```python
from build123d import *

# Parameters (mm, degrees)
F0_W     = 146.05
F0_H     = 114.3
F0_R     = 3.24
F0_W_2   = 5
F1_DEPTH = 50
F2_W     = 119.824
F2_H     = 108.7
F3_DEPTH = 45
F4_D     = 5.6
F4_DEPTH = 20
F4_TIP   = 1.6824097333
F5_W     = 40
F5_H     = 5
F6_DEPTH = 2.8
F7_D     = 4
F8_W     = 40
F8_H     = 10
F9_DEPTH = 50.001
F10_R    = 4


with BuildPart() as f1:
    # F0 (on Top) → F1 (new body)
    with BuildSketch(Plane.XY):
        Rectangle(F0_W, F0_H)
        with Locations((-68.262, -42.862)):
            Circle(F0_R, mode=Mode.SUBTRACT)
        with Locations((68.262, -42.862)):
            Circle(F0_R, mode=Mode.SUBTRACT)
        with Locations((-68.262, 4.763)):
            Circle(F0_R, mode=Mode.SUBTRACT)
        with BuildLine():
            Line((-72.225, -1.587), (-68.262, -1.587))
            ThreePointArc((-68.262, -1.587), (-61.912, 4.763), (-68.262, 11.113))
            Line((-68.262, 11.113), (-72.225, 11.113))
            Line((-72.225, 11.113), (-72.225, 36.512))
            Line((-72.225, 36.512), (-68.262, 36.512))
            ThreePointArc((-68.262, 36.512), (-61.912, 42.862), (-68.262, 49.212))
            Line((-68.262, 49.212), (-72.225, 49.212))
            Line((-72.225, 49.212), (-72.225, 56.35))
            Line((-72.225, 56.35), (72.225, 56.35))
            Line((72.225, 56.35), (72.225, 49.212))
            Line((72.225, 49.212), (68.262, 49.212))
            ThreePointArc((68.262, 49.212), (61.912, 42.862), (68.262, 36.512))
            Line((68.262, 36.512), (72.225, 36.512))
            Line((72.225, 36.512), (72.225, 11.113))
            Line((72.225, 11.113), (68.262, 11.113))
            ThreePointArc((68.262, 11.113), (61.912, 4.763), (68.262, -1.587))
            Line((68.262, -1.587), (72.225, -1.587))
            Line((72.225, -1.587), (72.225, -36.512))
            Line((72.225, -36.512), (68.262, -36.512))
            ThreePointArc((68.262, -36.512), (61.912, -42.862), (68.262, -49.212))
            Line((68.262, -49.212), (72.225, -49.212))
            Line((72.225, -49.212), (72.225, -56.35))
            Line((72.225, -56.35), (-72.225, -56.35))
            Line((-72.225, -56.35), (-72.225, -49.212))
            Line((-72.225, -49.212), (-68.262, -49.212))
            ThreePointArc((-68.262, -49.212), (-61.912, -42.862), (-68.262, -36.512))
            Line((-68.262, -36.512), (-72.225, -36.512))
            Line((-72.225, -36.512), (-72.225, -1.587))
        make_face(mode=Mode.SUBTRACT)
        with Locations((-68.262, 42.862)):
            Circle(F0_R, mode=Mode.SUBTRACT)
        with Locations((68.262, 4.763)):
            Circle(F0_R, mode=Mode.SUBTRACT)
        with Locations((68.262, 42.862)):
            Circle(F0_R, mode=Mode.SUBTRACT)
        with Locations((75.525, 0)):
            Rectangle(F0_W_2, F0_H)
        with Locations((-75.525, 0)):
            Rectangle(F0_W_2, F0_H)
        with Locations((-68.262, 4.763)):
            Circle(F0_R)
        with Locations((-68.262, 42.862)):
            Circle(F0_R)
        with Locations((68.262, 42.862)):
            Circle(F0_R)
        with BuildLine():
            ThreePointArc((-68.262, 11.113), (-61.912, 4.763), (-68.262, -1.587))
            Line((-68.262, -1.587), (-72.225, -1.587))
            Line((-72.225, -1.587), (-72.225, -36.512))
            Line((-72.225, -36.512), (-68.262, -36.512))
            ThreePointArc((-68.262, -36.512), (-61.912, -42.862), (-68.262, -49.212))
            Line((-68.262, -49.212), (-72.225, -49.212))
            Line((-72.225, -49.212), (-72.225, -56.35))
            Line((-72.225, -56.35), (72.225, -56.35))
            Line((72.225, -56.35), (72.225, -49.212))
            Line((72.225, -49.212), (68.262, -49.212))
            ThreePointArc((68.262, -49.212), (61.912, -42.862), (68.262, -36.512))
            Line((68.262, -36.512), (72.225, -36.512))
            Line((72.225, -36.512), (72.225, -1.587))
            Line((72.225, -1.587), (68.262, -1.587))
            ThreePointArc((68.262, -1.587), (61.912, 4.763), (68.262, 11.113))
            Line((68.262, 11.113), (72.225, 11.113))
            Line((72.225, 11.113), (72.225, 36.512))
            Line((72.225, 36.512), (68.262, 36.512))
            ThreePointArc((68.262, 36.512), (61.912, 42.862), (68.262, 49.212))
            Line((68.262, 49.212), (72.225, 49.212))
            Line((72.225, 49.212), (72.225, 56.35))
            Line((72.225, 56.35), (-72.225, 56.35))
            Line((-72.225, 56.35), (-72.225, 49.212))
            Line((-72.225, 49.212), (-68.262, 49.212))
            ThreePointArc((-68.262, 49.212), (-61.912, 42.862), (-68.262, 36.512))
            Line((-68.262, 36.512), (-72.225, 36.512))
            Line((-72.225, 36.512), (-72.225, 11.113))
            Line((-72.225, 11.113), (-68.262, 11.113))
        make_face()
        with Locations((68.262, 4.763)):
            Circle(F0_R)
        with Locations((68.262, -42.862)):
            Circle(F0_R)
        with Locations((-68.262, -42.862)):
            Circle(F0_R)
    extrude(amount=-F1_DEPTH)

    # F2 (on face) → F3 (cut)
    with BuildSketch(Plane.XY):
        Rectangle(F2_W, F2_H)
    extrude(amount=-F3_DEPTH, mode=Mode.SUBTRACT)

    # F4
    with Locations(Plane.XY):
        with Locations((-68.262, 42.862), (-68.262, 4.763), (-68.262, -42.862), (68.262, -42.862), (68.262, 4.763), (68.262, 42.862)):
            Hole(F4_D / 2, depth=F4_DEPTH)
            with Locations((0, 0, -(F4_DEPTH + F4_TIP / 2))):  # 118° drill point
                Cone(0, F4_D / 2, F4_TIP, mode=Mode.SUBTRACT)

    # F5 (on face) → F6 (cut, through all)
    with BuildSketch(Plane.XZ.offset(57.15)):
        with Locations((0, -42.5)):
            Rectangle(F5_W, F5_H)
    extrude(amount=-F6_DEPTH, mode=Mode.SUBTRACT)

    # F7 (through all)
    with Locations(Plane.XZ.offset(57.15)):
        with Locations((-49.912, -25), (49.912, -25)):
            Hole(F7_D / 2)

    # F8 (on face) → F9 (cut, through all)
    with BuildSketch(Plane.XY):
        with Locations((0, 49.35)):
            Rectangle(F8_W, F8_H)
    extrude(amount=-F9_DEPTH, mode=Mode.SUBTRACT)

    # F10
    f10_edges = [f1.edges().sort_by_distance(p)[0] for p in [
        (-20, 49.35, -45),
        (0, 44.35, -45),
        (20, 49.35, -45),
    ]]
    fillet(f10_edges, radius=F10_R)


solid = f1.part
```
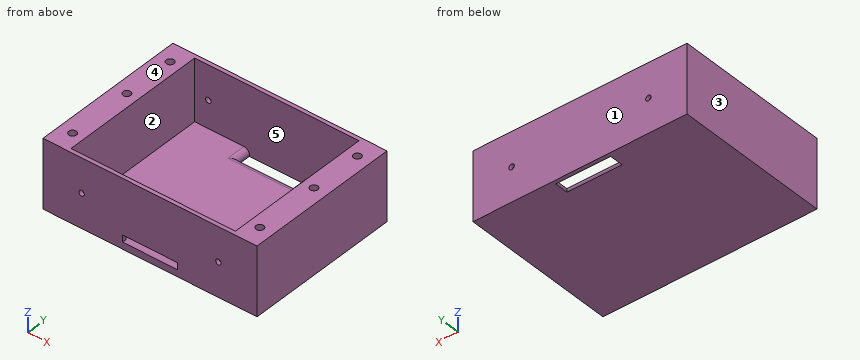
Geometry: final body of the model. Coordinates: model frame, mm. Face numbers are marked on the shaded views. A direction names the side the tool comes from. Coordinates: 2 decimals unless noted, no trailing zeros. Order: outer loops, then holes, each group sorted by start corner. A loop starts at its lowest first (then second) coordinate and runs counter-clockwise, first axis right, second up.
Item 1: Draft query along Y for the marked faces 1, 2 and 3. Return one class per face: released by +Y, released by -Y, zero draft, split by the parting line, or undercut.
Answer:
face 1: released by +Y
face 2: undercut
face 3: zero draft
Item 2: Section query C-C (z = -36.5). Output: boundary loops of the cut face in (x, y) (3 decimals).
Answer:
outline: (-78.025, -57.15) - (78.025, -57.15) - (78.025, 57.15) - (-78.025, 57.15) - close; hole (-59.912, -54.35) - (59.912, -54.35) - (59.912, 54.35) - (-59.912, 54.35) - close
Item 3: Section query D-D (y = -36). Output: boundary loops of the cut face in (x, z) (3 decimals).
Answer:
outline: (-78.025, -50) - (78.025, -50) - (78.025, 0) - (59.912, 0) - (59.912, -45) - (-59.912, -45) - (-59.912, 0) - (-78.025, 0) - close
Item 4: Access query for the marked faces 4 and 5. Directions: +Z, -Z, +X, -X, +Y, -Y. A direction counts if a zero-diameter tool reaches every point of the face in a straight line with its end or side. Return the directions, or none.
Answer:
face 4: +Z, +X, -X, +Y, -Y
face 5: +Z
Item 5: Section query B-B (x = -13). Output: boundary loops of the cut face in (y, z), then the cut area to 3 significant figures.
Answer:
outline: (-57.15, -50) - (44.35, -50) - (44.35, -49) arc R4 ccw to (40.35, -45) - (-57.15, -45) - close; (-57.15, -40) - (-54.35, -40) - (-54.35, 0) - (-57.15, 0) - close; (54.35, -50) - (57.15, -50) - (57.15, 0) - (54.35, 0) - close
area: 756 mm2
Item 6: Section query A-A (z = -25). Output: boundary loops of the cut face in (x, y) (3 decimals), then the cut area to 3 significant figures.
Answer:
outline: (-78.025, -57.15) - (-51.912, -57.15) - (-51.912, -54.35) - (-59.912, -54.35) - (-59.912, 54.35) - (-51.912, 54.35) - (-51.912, 57.15) - (-78.025, 57.15) - close; (-47.912, -57.15) - (47.912, -57.15) - (47.912, -54.35) - (-47.912, -54.35) - close; (-47.912, 54.35) - (47.912, 54.35) - (47.912, 57.15) - (-47.912, 57.15) - close; (51.912, -57.15) - (78.025, -57.15) - (78.025, 57.15) - (51.912, 57.15) - (51.912, 54.35) - (59.912, 54.35) - (59.912, -54.35) - (51.912, -54.35) - close
area: 4,770 mm2
Item 7: Material intervals for line 1 along X through (y, z) = (34.5, -18) (3 decimals); line 2 along Y through (x, z) = (-39, -17.5); line 3 along Y through (x, z) = (66, -13.5), sorted ascending.
Answer:
line 1: x = -78.025 to -59.912, 59.912 to 78.025
line 2: y = -57.15 to -54.35, 54.35 to 57.15
line 3: y = -57.15 to -44.51, -41.21 to 3.11, 6.41 to 41.21, 44.51 to 57.15
